CAD build for the part. Positions are in the model's coordinates, mm. Give positions to 0.01 mm unless a question says otherwise; leave off trailing zeros. Loops run counter-clockwise (first coordinate to the right, second up) from the corner with the lowest first, then second, coordinate; pieces in that order, holes last. Notation, with made-up numbers: M -0.5,26 L 15.5,26 A18 ccw 15.5,36 Z; hole C -26.75,54 d5. An arc over 180 degrees is marked long. One line per question, with ' | ' between items.
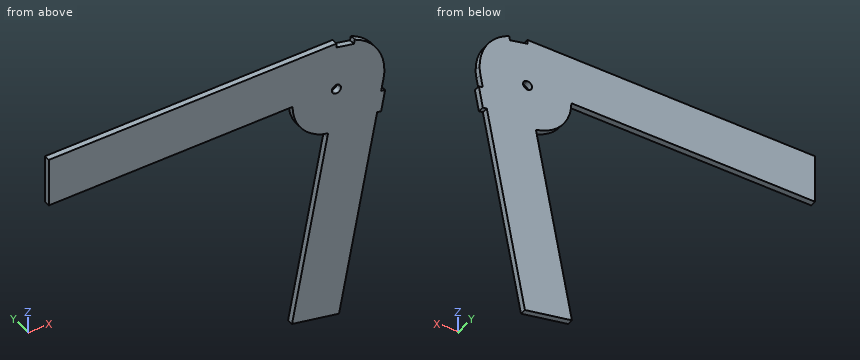
```python
from build123d import *

# Parameters (mm, degrees)
F1_DEPTH = 6.35


with BuildPart() as f1:
    # F0 (on Front) → F1 (new body)
    with BuildSketch(Plane.XZ):
        with BuildLine():
            ThreePointArc((-50.8, 0), (-35.9210244843, 35.9210244843), (0, 50.8))
            Line((0, 50.8), (-304.8, 50.8))
            Line((-304.8, 50.8), (-304.8, 0))
            Line((-304.8, 0), (-50.8, 0))
        make_face()
        Polygon((51.6320080606, -22.9739477141), (46.3118022943, -27.9812591796), (43.1772616128, -44.1070730311), (47.3658829955, -44.9212585503), align=None)
        Polygon((51.6320080606, -22.9739477141), (47.4433866779, -22.1597621949), (46.3118022943, -27.9812591796), align=None)
        with BuildLine():
            Line((46.482, 0), (50.8, 0))
            ThreePointArc((50.8, 0), (42.2710462755, 28.1744325014), (19.5480847725, 46.8882968525))
            Line((19.5480847725, 46.8882968525), (18.6457425678, 42.5783114754))
            ThreePointArc((18.6457425678, 42.5783114754), (38.905447755, 25.4350635734), (46.482, 0))
        make_face()
        with BuildLine():
            Line((47.4433866779, -22.1597621949), (49.8666609191, -9.6930969651))
            ThreePointArc((49.8666609191, -9.6930969651), (28.4069994963, -42.1151086858), (-9.6930969651, -49.8666609191))
            Line((-9.6930969651, -49.8666609191), (-47.0680440019, -242.1440947937))
            Line((-47.0680440019, -242.1440947937), (2.7986169173, -251.8371917588))
            Line((2.7986169173, -251.8371917588), (43.1772616128, -44.1070730311))
            Line((43.1772616128, -44.1070730311), (46.3118022943, -27.9812591796))
            Line((46.3118022943, -27.9812591796), (47.4433866779, -22.1597621949))
        make_face()
        with BuildLine():
            ThreePointArc((49.8666609191, -9.6930969651), (50.5661268771, -4.868964228), (50.8, 0))
            Line((50.8, 0), (46.482, 0))
            ThreePointArc((46.482, 0), (46.2680060925, -4.4551022686), (45.627994741, -8.8691837231))
            Line((45.627994741, -8.8691837231), (49.8666609191, -9.6930969651))
        make_face()
        with BuildLine():
            Line((0, 46.482), (0, 50.8))
            ThreePointArc((0, 50.8), (-35.9210244843, 35.9210244843), (-50.8, 0))
            Line((-50.8, 0), (-46.482, 0))
            ThreePointArc((-46.482, 0), (-32.8677374031, 32.8677374031), (0, 46.482))
        make_face()
        with BuildLine():
            ThreePointArc((-9.6930969651, -49.8666609191), (28.4069994963, -42.1151086858), (49.8666609191, -9.6930969651))
            Line((49.8666609191, -9.6930969651), (45.627994741, -8.8691837231))
            ThreePointArc((45.627994741, -8.8691837231), (25.9924045391, -38.5353244475), (-8.8691837231, -45.627994741))
            Line((-8.8691837231, -45.627994741), (-9.6930969651, -49.8666609191))
        make_face()
        with BuildLine():
            Line((4.7625, 0), (46.482, 0))
            ThreePointArc((46.482, 0), (38.905447755, 25.4350635734), (18.6457425678, 42.5783114754))
            Line((18.6457425678, 42.5783114754), (0, 46.482))
            Line((0, 46.482), (0, 4.7625))
            ThreePointArc((0, 4.7625), (0.4564653964, 4.7405743947), (0.9087278405, 4.6749994612))
            ThreePointArc((0.9087278405, 4.6749994612), (3.6748620784, 3.0293225241), (4.7625, 0))
        make_face()
        with BuildLine():
            Line((0, 4.7625), (0, 46.482))
            ThreePointArc((0, 46.482), (-32.8677374031, 32.8677374031), (-46.482, 0))
            Line((-46.482, 0), (-4.7625, 0))
            ThreePointArc((-4.7625, 0), (-3.3675960454, 3.3675960454), (0, 4.7625))
        make_face()
        with BuildLine():
            ThreePointArc((-46.482, 0), (-35.866653885, -29.566187835), (-8.8691837231, -45.627994741))
            Line((-8.8691837231, -45.627994741), (-0.9087278405, -4.6749994612))
            ThreePointArc((-0.9087278405, -4.6749994612), (-3.6748620784, -3.0293225241), (-4.7625, 0))
            Line((-4.7625, 0), (-46.482, 0))
        make_face()
        with BuildLine():
            ThreePointArc((-8.8691837231, -45.627994741), (25.9924045391, -38.5353244475), (45.627994741, -8.8691837231))
            Line((45.627994741, -8.8691837231), (4.6749994612, -0.9087278405))
            ThreePointArc((4.6749994612, -0.9087278405), (2.6631562028, -3.9482914393), (-0.9087278405, -4.6749994612))
            Line((-0.9087278405, -4.6749994612), (-8.8691837231, -45.627994741))
        make_face()
        with BuildLine():
            ThreePointArc((45.627994741, -8.8691837231), (46.2680060925, -4.4551022686), (46.482, 0))
            Line((46.482, 0), (4.7625, 0))
            ThreePointArc((4.7625, 0), (4.7405743947, -0.4564653964), (4.6749994612, -0.9087278405))
            Line((4.6749994612, -0.9087278405), (45.627994741, -8.8691837231))
        make_face()
    extrude(amount=F1_DEPTH)


solid = f1.part
```
Item 1: Saw through at A-A on x = -14. Give the cut face in (y, z), and give its area (3 significant figures).
Conclusion:
outline: M -6.35,-248.57 L 0,-248.57 L 0,-72.02 L -6.35,-72.02 Z; M -6.35,-44.32 L 0,-44.32 L 0,50.8 L -6.35,50.8 Z | area: 1,730 mm²
Item 2: Saw through at D-D on z = 32. Give the cut face in (x, y), and give its area (3 significant figures).
Conclusion:
outline: M -304.8,-6.35 L 39.45,-6.35 L 39.45,0 L -304.8,0 Z | area: 2,190 mm²
Item 3: Drop flat-ended pins along their axis: P1, Ø1, axis at x = -159, y = -4.5, coming from the -Z side; P2, Ø2, axis at y = -5, z = -65, coming from the +X side. Give the stop position or say it passes through.
Conclusion:
P1: z = 0 | P2: x = 39.31
Item 4: Saw through at B-B on y = -4.5. Give the cut face in (x, z) (1 decimal), and give its area (3 significant figures).
Conclusion:
outline: M -304.8,0 L -46.5,0 A46.5 ccw -8.9,-45.6 L -47.1,-242.1 L 2.8,-251.8 L 43.2,-44.1 L 47.4,-44.9 L 51.6,-23 L 47.4,-22.2 L 49.9,-9.7 A50.8 ccw 19.5,46.9 L 18.6,42.6 L 0,46.5 L 0,50.8 L -304.8,50.8 Z; hole C 0,0 d9.5 | area: 31,700 mm²
Item 5: Saw through at C-C on x = -101. Give the cut face in (y, z).
Conclusion:
outline: M -6.35,0 L 0,0 L 0,50.8 L -6.35,50.8 Z
Item 6: Drill centre lines: line 1 along Z through (x, y) = (-194, -3.5); line 2 along X through (y, z) = (-1, 18); line 3 along Z through (x, y) = (-3.5, -0.25). Where is each one in solid material? Low to high. Write a range as [from, to].
Conclusion:
line 1: [0, 50.8] | line 2: [-304.8, 47.5] | line 3: [-250.61, -3.23], [3.23, 50.8]
